Answer from the drawing. Dimensions are ordinates in mm from the lowest x, y and z of the part. Coordinates: 2 decimals unless noted, no trailing zeros. Order: outer loops, then holes, each group sorted by start corner. A loop starts at its lowest first (then second) coordinate and runs counter-clockwise, first axis right, second up. Notation, with made-up numbers: (64, 29.25) -> (69, 29.25) arc R19 ccw to (69, 54.25) -> close; hole circle Ø5 at (-12, 5.25). An arc over 180 degrees is marked (long way). Answer as a JSON object with one key per item and string values. Group by question number.
1) Section C-C on z = 126.5 is taken. Determine the outline of the cut face in (x, y).
2) Consider L1, parallel to Y at x = 85, z = 144; L2, parallel to X at y = 10, z = 119; L3, parallel to X at y = 157.5, z = 20. Determine where each line is inside the solid, lowest interval first.
3) Section B-B on x = 85 is taken. Determine the outline of the cut face in (y, z), and give its area (3 significant figures).
4) Section A-A on y = 85 is taken. Determine the outline of the cut face in (x, z).
5) Given pin 1 (3 mm diameter, centred on x = 60, z = 24.5, fed in from +Y); pin 2 (3 mm diameter, centred on x = 84.5, z = 123, fed in from +Y); pin 3 (5 mm diameter, centred on x = 42.5, z = 31, fed in from -Y), each flat-ended and moving along its own axis, determine where each tip first touches the part or whether it passes through.
6) Section D-D on z = 20 is taken. Determine the outline of the cut face in (x, y).
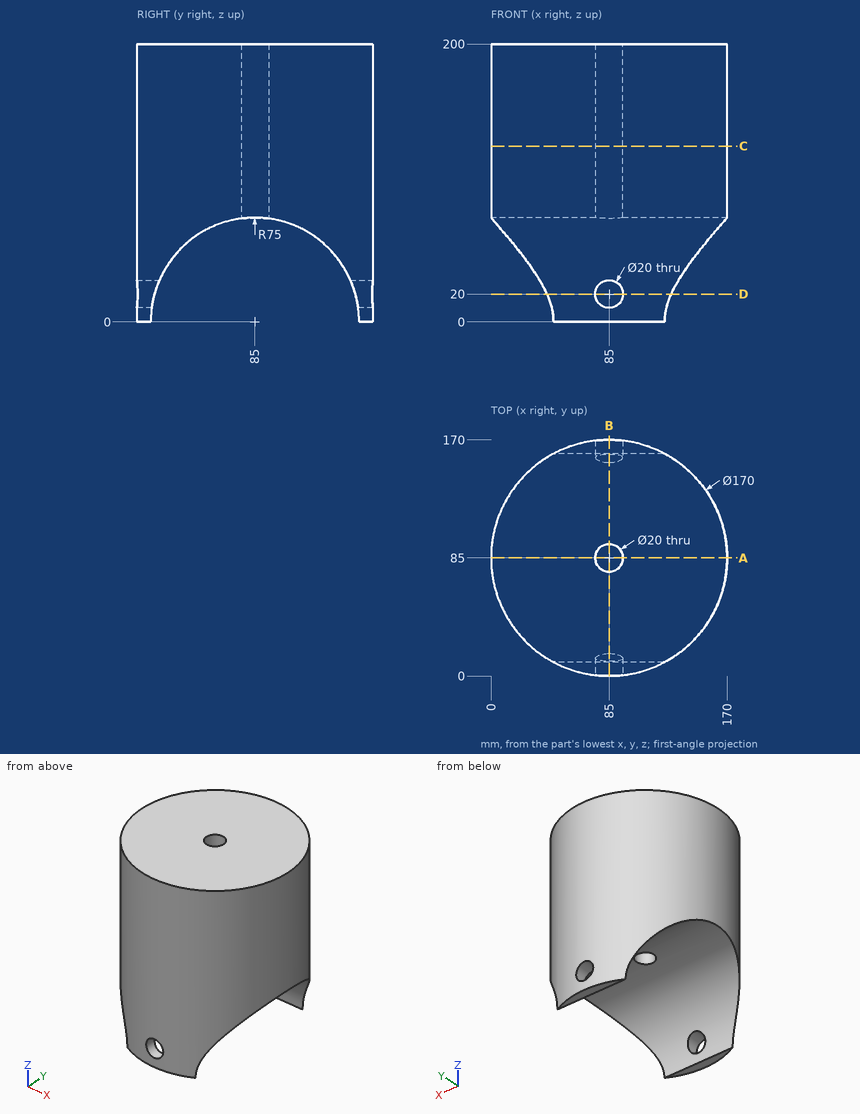
Worked answers:
{
 "1": {"outline": "circle Ø170 at (85, 85); hole circle Ø20 at (85, 85)"},
 "2": {"L1": "y = 0 to 75, 95 to 170", "L2": "x = 45 to 125", "L3": "x = 40.63 to 75, 95 to 129.37"},
 "3": {"outline": "(0, 0) -> (10, 0) arc R75 cw to (10.67, 10) -> (0, 10) -> close; (0, 30) -> (16.26, 30) arc R75 cw to (75, 74.33) -> (75, 200) -> (0, 200) -> close; (95, 74.33) arc R75 cw to (153.74, 30) -> (170, 30) -> (170, 200) -> (95, 200) -> close; (159.33, 10) arc R75 cw to (160, 0) -> (170, 0) -> (170, 10) -> close", "area": "22,100 mm²"},
 "4": {"outline": "(0, 75) -> (75, 75) -> (75, 200) -> (0, 200) -> close; (95, 75) -> (170, 75) -> (170, 200) -> (95, 200) -> close"},
 "5": {"pin 1": "stops at y = 166.69", "pin 2": "stops at y = 170", "pin 3": "stops at y = 10"},
 "6": {"outline": "(40.28, 12.72) arc R85 ccw to (75, 0.59) -> (75, 12.72) -> close; (40.28, 157.28) -> (75, 157.28) -> (75, 169.41) arc R85 ccw to start; (95, 0.59) arc R85 ccw to (129.72, 12.72) -> (95, 12.72) -> close; (95, 157.28) -> (129.72, 157.28) arc R85 ccw to (95, 169.41) -> close"}
}
